Here's how the part is built. I have some questions about the finished solid (model axes, mm). Coordinates: 2 decimals unless noted, no trailing zeros. Write each loop counter-clockwise with the first axis right and the second up, starting at its lowest first coordinate (ties: lowest second). Pieces come first, ordered by that corner, then holes.
(1) Imagine slicing it at A-A, the plane x = 0. List the corners of the cut face in (y, z) for me, plus the area to 3 significant figures.
(2) Imagine slicing it at B-B, the plane z = 419.5. List the corners of the cut face in (x, y) for me.
(3) For pin 1 Ø1.5 at (x, y) = (-2.5, -1) entering from -Z; pin 2 Ø1 at (x, z) = (-2, 507.5) entering from +Y; pin 3 Ø5 at (y, z) = (0, 63) entering from -X, each with a flat end and sliding along its axis, tell me the tip position at first contact or that it passes through.
(4) Please list where these lines run through material, in increasing order: probe 1 along Z at (x, y) = (0, -4.65); probe 2 along Z at (x, y) = (4.55, 0); probe 3 along Y at (x, z) = (0, 47).
```python
from build123d import *

# Parameters (mm, degrees)
SKETCH_1_R               = 5
SKETCH_1_R_2             = 4
EXTRUDE_1_DEPTH          = 676.5
CUT_EXTRUDE_1_DEPTH      = 677.536953906
CUT_EXTRUDE_1_DEPTH_BACK = 677.536953906
SKETCH_2_R               = 2
SKETCH_2_R_2             = 1.5
SKETCH_2_3_R             = 4
SKETCH_2_3_R_2           = 3
CUT_EXTRUDE_2_DEPTH      = 677.536954007
CUT_EXTRUDE_3_DEPTH      = 677.536954007
CUT_EXTRUDE_3_DEPTH_BACK = 677.536954007
SKETCH_3_R               = 1.5
SKETCH_3_3_R             = 3
CUT_EXTRUDE_4_DEPTH      = 10


with BuildPart() as part:
    # Sketch 1 → Extrude 1 (new body)
    with BuildSketch(Plane.XY):
        Circle(SKETCH_1_R)
        Circle(SKETCH_1_R_2, mode=Mode.SUBTRACT)
    extrude(amount=EXTRUDE_1_DEPTH)

    # Sketch 2 → Cut-Extrude 1 (cut, two sides: drawn at the far end of the back side and taken through both)
    with BuildSketch(Plane(origin=(0, 0, 0), x_dir=(1, 0, 0), z_dir=(0, 1, 0)).offset(-CUT_EXTRUDE_1_DEPTH_BACK)):
        with Locations(Location((0, -660.5, 0), (0, 0, 270))):
            Circle(SKETCH_2_R)
        with Locations(Location((0, -637.5, 0), (0, 0, 270))):
            Circle(SKETCH_2_R_2)
    extrude(amount=CUT_EXTRUDE_1_DEPTH + CUT_EXTRUDE_1_DEPTH_BACK, mode=Mode.SUBTRACT)

    # Sketch 2_3 → Cut-Extrude 2 (cut, through all)
    with BuildSketch(Plane(origin=(0, 0, 0), x_dir=(1, 0, 0), z_dir=(0, 1, 0))):
        with Locations(Location((0, -660.5, 0), (0, 0, 90))):
            Circle(SKETCH_2_3_R)
        with Locations(Location((0, -637.5, 0), (0, 0, 90))):
            Circle(SKETCH_2_3_R_2)
    extrude(amount=CUT_EXTRUDE_2_DEPTH, mode=Mode.SUBTRACT)

    # Sketch 3 → Cut-Extrude 3 (cut, two sides: drawn at the far end of the back side and taken through both)
    with BuildSketch(Plane(origin=(0, 0, 0), x_dir=(0, 0, -1), z_dir=(1, 0, 0)).offset(-CUT_EXTRUDE_3_DEPTH_BACK)):
        with Locations((-63, 0)):
            Circle(SKETCH_3_R)
    extrude(amount=CUT_EXTRUDE_3_DEPTH + CUT_EXTRUDE_3_DEPTH_BACK, mode=Mode.SUBTRACT)

    # Sketch 3_3 → Cut-Extrude 4 (cut)
    with BuildSketch(Plane(origin=(0, 0, 0), x_dir=(0, 0, -1), z_dir=(1, 0, 0))):
        with Locations(Location((-63, 0, 0), (0, 0, 180))):
            Circle(SKETCH_3_3_R)
    extrude(amount=-CUT_EXTRUDE_4_DEPTH, mode=Mode.SUBTRACT)


solid = part.part
```
Recorded:
1. outline: (-5, 0) - (-4, 0) - (-4, 636) - (-5, 636) - close; (-5, 639) - (-4, 639) - (-4, 658.5) - (-5, 658.5) - close; (-5, 662.5) - (-4, 662.5) - (-4, 676.5) - (-5, 676.5) - close; (4, 0) - (5, 0) - (5, 634.5) - (4, 634.5) - close; (4, 640.5) - (5, 640.5) - (5, 656.5) - (4, 656.5) - close; (4, 664.5) - (5, 664.5) - (5, 676.5) - (4, 676.5) - close
1. area: 1,330 mm2
2. outline: circle Ø10 at (0, 0); hole circle Ø8 at (0, 0)
3. pin 1: passes through
3. pin 2: stops at y = 4.77
3. pin 3: stops at x = 3.12
4. probe 1: z = 0 to 636, 639 to 658.5, 662.5 to 676.5
4. probe 2: z = 0 to 61.5, 64.5 to 676.5
4. probe 3: y = -5 to -4, 4 to 5
